```python
from build123d import *

# Parameters (mm, degrees)
F0_R     = 2.1
F1_DEPTH = 4
F2_W     = 7
F2_H     = 30
F3_DEPTH = 20
F5_W     = 5
F5_H     = 30
F6_DEPTH = 5
F7_SIZE  = 4.99999
F4_W     = 12
F4_H     = 6.2
F8_DEPTH = 10.8
F9_R     = 5


# Not quite as in the source:
# - a fillet or chamfer is up to 0.001 mm smaller than in the source, because OpenCascade refuses the exact size


with BuildPart() as f1:
    # F0 (on Front) → F1 (new body)
    with BuildSketch(Plane.XZ):
        with BuildLine():
            Line((55, 15), (-40, 15))
            ThreePointArc((-40, 15), (-43.5355339059, 13.5355339059), (-45, 10))
            Line((-45, 10), (-45, -10))
            ThreePointArc((-45, -10), (-43.5355339059, -13.5355339059), (-40, -15))
            Line((-40, -15), (55, -15))
            Line((55, -15), (55, 15))
        make_face()
        with Locations((-25, 0)):
            Circle(F0_R, mode=Mode.SUBTRACT)
        with Locations((25, 0)):
            Circle(F0_R, mode=Mode.SUBTRACT)
    extrude(amount=F1_DEPTH)

    # F2 (on face) → F3 (join)
    with BuildSketch(Plane.XZ.offset(4)):
        with Locations((51.5, 0)):
            Rectangle(F2_W, F2_H)
    extrude(amount=F3_DEPTH)

    # F5 (on face) → F6 (join)
    with BuildSketch(Plane.XZ.offset(4)):
        with Locations((45.5, 0)):
            Rectangle(F5_W, F5_H)
    extrude(amount=F6_DEPTH)

    # F7 (size 5 in the source; OpenCascade refuses exactly that, so slightly less here)
    f7_edges = [f1.edges().sort_by_distance(p)[0] for p in [
        (43, -9, 0),
    ]]
    chamfer(f7_edges, length=F7_SIZE)

    # F4 (on face) → F8 (cut, symmetric)
    with BuildSketch(Plane(origin=(48, 0, 0), x_dir=(0, -1, 0), z_dir=(-1, 0, 0))):
        with Locations((14, 0)):
            Rectangle(F4_W, F4_H)
    extrude(amount=F8_DEPTH, both=True, mode=Mode.SUBTRACT)

    # F9
    f9_edges = [f1.edges().sort_by_distance(p)[0] for p in [
        (51.5, -24, 15),
        (51.5, -24, -15),
    ]]
    fillet(f9_edges, radius=F9_R)


solid = f1.part
```
Design review of the part built by this model. Coordinates are the model's own, in mm. A direction names the side the tool comes from. Give positions to 0.01 mm unless a question says otherwise; leave off trailing zeros. Order: outer loops, then holes, each group sorted by start corner. A loop starts at its lowest first (then second) coordinate and runs counter-clockwise, first axis right, second up. Notation, with made-up numbers: (17, -32) -> (49, -32) arc R18 ccw to (49, -10) -> close; hole circle Ø9 at (4, 73.25). An arc over 180 degrees is marked (long way). Write item = value, one per line. Start each with the question number.
(1) For pin 1 (4 mm diameter, centred on y = -11.5, z = -8, fed in from -X); pin 2 (6.5 mm diameter, centred on x = -25, z = 0, fed in from -Y), all flat-tipped, find the tip position at first contact; note any pin that passes through.
(2) To check wall thickness, follow line 1 along Z through (x, y) = (-25, -1.6); line 2 along X through (y, z) = (-14.5, 6); line 3 along Y through (x, z) = (-4.5, -12). State the ranges of each line that lie inside material, in increasing order.
(3) For faces 1 (the face through (52, -14, 3.1)), 2 (the face through (18, -3, 15)), 3 (the face through (48, -16, -4)), list the 3-axis set-ups (+Z, -Z, +X, -X, +Y, -Y) from which the entire face can be reached by the end or side of a thin tool; tool diameter is ignored.
(4) We need section A-A on x = 49. Write out the cut boundary in (y, z), plus the area to 3 significant figures.
(5) Mouldability with a two-part tool opening along Y and no side actions: class faces 4 (the face through (-22.997, -1.972, 0.631)), 5 (the face through (-2, -4, 0)), 6 (the face through (4, 0, 0)), 7 (the face through (51, -20, 0)) as +Y half, -Y half, draft (parallel to the pull), parting line (faces both ways), or undercut.
(6) We need section C-C on y = -16.5. Write out the cut boundary in (x, z).
(7) We need section B-B on z = 0. State how many separate pieces and enclosed holes the cut face has, plus the area to 3 significant figures.
(8) We need section D-D on x = 25. Write out the cut boundary in (y, z), plus the area to 3 significant figures.
Numbers:
q1.pin_1 = 48
q1.pin_2 = -4
q2.line_1 = -15 to -2.1, 2.1 to 15
q2.line_2 = 48 to 55
q2.line_3 = -4 to 0
q3.face_1 = +X, -X
q3.face_2 = +Z, +X, -X, +Y, -Y
q3.face_3 = +Z, -Z, -X, -Y
q4.outline = (-24, -10) arc R5 ccw to (-19, -15) -> (0, -15) -> (0, 15) -> (-19, 15) arc R5 ccw to (-24, 10) -> close; hole (-20, -3.1) -> (-8, -3.1) -> (-8, 3.1) -> (-20, 3.1) -> close
q4.area = 635 mm^2
q5.face_4 = draft
q5.face_5 = -Y half
q5.face_6 = +Y half
q5.face_7 = undercut
q6.outline = (48, -15) -> (55, -15) -> (55, -3.1) -> (48, -3.1) -> close; (48, 3.1) -> (55, 3.1) -> (55, 15) -> (48, 15) -> close
q7.separate_pieces = 4
q7.enclosed_holes = 0
q7.area = 434 mm^2
q8.outline = (-4, -15) -> (0, -15) -> (0, -2.1) -> (-4, -2.1) -> close; (-4, 2.1) -> (0, 2.1) -> (0, 15) -> (-4, 15) -> close
q8.area = 103 mm^2
